CAD build for the part. Positions are in the model's coordinates, mm. Face numbers are marked on the shaded views. A direction names the side the tool comes from. Coordinates: 2 decimals unless noted, no trailing zeros. Loops run counter-clockwise (first coordinate to the right, second up) from the corner with the lowest first, then second, coordinate; pieces in that order, holes last.
1) Saw through at C-C, the plane y = 12.5. Write the cut outline in (x, z), and give its area (3 significant figures).
2) Pin check, flat tips, straight feed: pin 1 Ø1.9 at (x, z) = (7, 0) entering from -Y (1 decimal); pin 2 Ø3 at (x, y) = (8.5, 3.5) entering from -Z; pin 3 Ø5 at (x, y) = (-7, 9.5) entering from +Z; pin 4 Ø6 at (y, z) = (12, 4) entering from -X. Stop position of each tip, or through.
3) Two-plate mould, pull along Z, no slides. Class the marked faces 1, 2 and 3: +Z half, -Z half, draft (parallel to the pull), parting line (faces both ways), or undercut.
4) Saw through at D-D, the plane z = -2.75. Write the cut outline in (x, y), and give its area (3 significant figures).
5) Saw through at A-A, the plane z = 0. Give the number of separate pieces and of enclosed holes in the cut face, and give its area (3 significant figures).
6) Which spindle directions (+Z, -Z, +X, -X, +Y, -Y) get a long thin tool onto all of the face, cutting with end or side? Do the marked faces 4, 5 and 6. Say none if no direction does.
7) Wall check: line 1 along X through (y, z) = (2.1, 0); line 2 along X through (y, z) = (-0.25, 0); line 3 along Y through (x, z) = (3, -8.75). Give the ranges that are in metal, low to high.
8) Saw through at B-B, the plane x = 7. Write the cut outline in (y, z), and give its area (3 significant figures).
```python
from build123d import *

# Parameters (mm, degrees)
SKETCH_1_R          = 10.85
SKETCH_1_R_2        = 3.4
EXTRUDE_1_DEPTH     = 3.5
SKETCH_2_R          = 5
SKETCH_2_R_2        = 3.35
EXTRUDE_2_DEPTH     = 10
SKETCH_3_R          = 1.6
CUT_EXTRUDE_1_DEPTH = 19.315157657
EXTRUDE_START       = 1.5
SKETCH_4_R          = 5
SKETCH_4_R_2        = 3.35
EXTRUDE_3_DEPTH     = 1.5


with BuildPart() as part:
    # Эскиз1 → Бобышка-Вытянуть1 (new body)
    with BuildSketch(Plane(origin=(0, 0, 0), x_dir=(1, 0, 0), z_dir=(0, 1, 0))):
        with Locations(Location((0, 0, 0), (0, 0, 270))):
            Circle(SKETCH_1_R)
        with Locations(Location((0, 0, 0), (0, 0, 270))):
            Circle(SKETCH_1_R_2, mode=Mode.SUBTRACT)
    extrude(amount=EXTRUDE_1_DEPTH)

    # Эскиз2 → Бобышка-Вытянуть2 (add)
    with BuildSketch(Plane(origin=(0, 3.5, 0), x_dir=(1, 0, 0), z_dir=(0, 1, 0))):
        with Locations(Location((0, 0, 0), (0, 0, 270))):
            Circle(SKETCH_2_R)
        with Locations(Location((0, 0, 0), (0, 0, 270))):
            Circle(SKETCH_2_R_2, mode=Mode.SUBTRACT)
    extrude(amount=EXTRUDE_2_DEPTH)

    # Эскиз3 → Вырез-Вытянуть1 (cut, through all)
    with BuildSketch(Plane(origin=(0, 3.5, 0), x_dir=(1, 0, 0), z_dir=(0, 1, 0))):
        with Locations(Location((0, 7, 0), (0, 0, 270))):
            Circle(SKETCH_3_R)
        with Locations(Location((-7, 0, 0), (0, 0, 270))):
            Circle(SKETCH_3_R)
        with Locations(Location((0, -7, 0), (0, 0, 270))):
            Circle(SKETCH_3_R)
        with Locations(Location((7, 0, 0), (0, 0, 270))):
            Circle(SKETCH_3_R)
    extrude(amount=-CUT_EXTRUDE_1_DEPTH, mode=Mode.SUBTRACT)

    # Эскиз4 → Бобышка-Вытянуть3 (add)
    with BuildSketch(Plane(origin=(0, 0, 0), x_dir=(-1, 0, 0), z_dir=(0, -1, 0)).offset(EXTRUDE_START)):
        with Locations(Location((0, 0, 0), (0, 0, 270))):
            Circle(SKETCH_4_R)
        with Locations(Location((0, 0, 0), (0, 0, 270))):
            Circle(SKETCH_4_R_2, mode=Mode.SUBTRACT)
    extrude(amount=-EXTRUDE_3_DEPTH)


solid = part.part
```
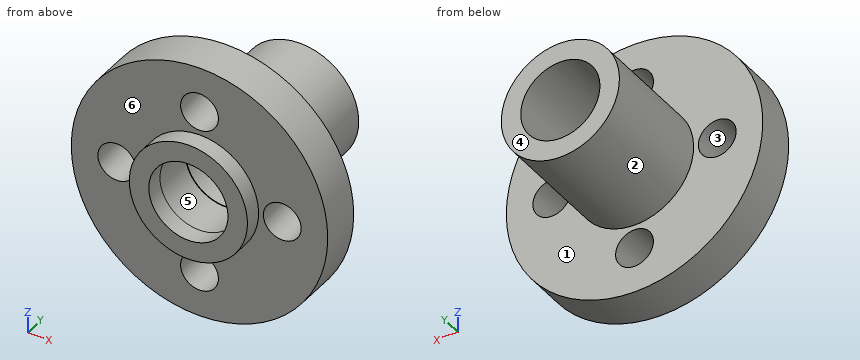
Data:
1. outline: circle Ø10 at (0, 0); hole circle Ø6.7 at (0, 0)
1. area: 43.3 mm2
2. pin 1: passes through
2. pin 2: stops at z = -8.29
2. pin 3: stops at z = 2.18
2. pin 4: stops at x = -4.9
3. face 1: draft
3. face 2: parting line
3. face 3: undercut
4. outline: (-10.5, 0) - (-4.18, 0) - (-4.18, -1.5) - (-1.91, -1.5) - (-1.91, 0) - (-2, 0) - (-2, 3.5) - (-1.91, 3.5) - (-1.91, 13.5) - (-4.18, 13.5) - (-4.18, 3.5) - (-10.5, 3.5) - close; (1.91, -1.5) - (4.18, -1.5) - (4.18, 0) - (10.5, 0) - (10.5, 3.5) - (4.18, 3.5) - (4.18, 13.5) - (1.91, 13.5) - (1.91, 3.5) - (2, 3.5) - (2, 0) - (1.91, 0) - close
4. area: 112 mm2
5. separate pieces: 4
5. enclosed holes: 0
5. area: 67.7 mm2
6. face 4: +Z, -Z, +X, -X, +Y
6. face 5: none
6. face 6: -Y
7. line 1: x = -10.85 to -8.6, -5.4 to -3.4, 3.4 to 5.4, 8.6 to 10.85
7. line 2: x = -5 to -3.35, 3.35 to 5
7. line 3: y = 0 to 3.5
8. outline: (0, -8.29) - (3.5, -8.29) - (3.5, -1.6) - (0, -1.6) - close; (0, 1.6) - (3.5, 1.6) - (3.5, 8.29) - (0, 8.29) - close
8. area: 46.8 mm2
